```python
from build123d import *

# Parameters (mm, degrees)
BOSS_EXTRUDE1_DEPTH = 2
CUT_EXTRUDE1_REACH  = 186.662
SKETCH3_W           = 25
SKETCH3_H           = 4
CUT_EXTRUDE2_DEPTH  = 185.661853126
SKETCH4_W           = 4
SKETCH4_H           = 10
BOSS_EXTRUDE2_DEPTH = 4


with BuildPart() as part:
    # Sketch1 → Boss-Extrude1 (new, symmetric)
    with BuildSketch(Plane.XY):
        Polygon((0, 4), (0, 72), (-170, 72), (-35, 19), (-35, 4), align=None)
    extrude(amount=BOSS_EXTRUDE1_DEPTH, both=True)

    # Sketch2 → Cut-Extrude1 (cut, up to next)
    with BuildSketch(Plane.XY.offset(2), mode=Mode.PRIVATE) as cut_extrude1_sk1:
        with BuildLine():
            Line((-3, 11), (-3, 7.5))
            ThreePointArc((-3, 7.5), (-4.5, 6), (-6, 7.5))
            Line((-6, 7.5), (-6, 11))
            ThreePointArc((-6, 11), (-4.5, 12.5), (-3, 11))
        make_face()
    cut_extrude1_tool1 = extrude(cut_extrude1_sk1.sketch, amount=-CUT_EXTRUDE1_REACH, mode=Mode.PRIVATE) & part.part
    # Sketch2 → Cut-Extrude1 (cut, up to next)
    with BuildSketch(Plane.XY.offset(2), mode=Mode.PRIVATE) as cut_extrude1_sk2:
        with BuildLine():
            Line((-32, 11), (-32, 7.5))
            ThreePointArc((-32, 7.5), (-30.5, 6), (-29, 7.5))
            Line((-29, 7.5), (-29, 11))
            ThreePointArc((-29, 11), (-30.5, 12.5), (-32, 11))
        make_face()
    cut_extrude1_tool2 = extrude(cut_extrude1_sk2.sketch, amount=-CUT_EXTRUDE1_REACH, mode=Mode.PRIVATE) & part.part
    add(cut_extrude1_tool1.solids().sort_by_distance((-4.5, 9.25, 2))[0], mode=Mode.SUBTRACT)
    add(cut_extrude1_tool2.solids().sort_by_distance((-30.5, 9.25, 2))[0], mode=Mode.SUBTRACT)

    # Sketch3 → Cut-Extrude2 (cut, through all)
    with BuildSketch(Plane.XY.offset(2)):
        with Locations((-62.5, 70)):
            Rectangle(SKETCH3_W, SKETCH3_H)
        with Locations((-12.5, 70)):
            Rectangle(SKETCH3_W, SKETCH3_H)
        with Locations((-112.5, 70)):
            Rectangle(SKETCH3_W, SKETCH3_H)
        with Locations((-162.5, 70)):
            Rectangle(SKETCH3_W, SKETCH3_H)
        with Locations((-212.5, 70)):
            Rectangle(SKETCH3_W, SKETCH3_H)
        with Locations((-262.5, 70)):
            Rectangle(SKETCH3_W, SKETCH3_H)
        with Locations((-312.5, 70)):
            Rectangle(SKETCH3_W, SKETCH3_H)
        with Locations((-362.5, 70)):
            Rectangle(SKETCH3_W, SKETCH3_H)
        with Locations((-412.5, 70)):
            Rectangle(SKETCH3_W, SKETCH3_H)
        with Locations((-462.5, 70)):
            Rectangle(SKETCH3_W, SKETCH3_H)
    extrude(amount=-CUT_EXTRUDE2_DEPTH, mode=Mode.SUBTRACT)

    # Sketch4 → Boss-Extrude2 (add)
    with BuildSketch(Plane(origin=(0, 0, 0), x_dir=(0, 0, -1), z_dir=(1, 0, 0))):
        with Locations((0, 63)):
            Rectangle(SKETCH4_W, SKETCH4_H)
        with Locations((0, 38)):
            Rectangle(SKETCH4_W, SKETCH4_H)
        with Locations((0, 13)):
            Rectangle(SKETCH4_W, SKETCH4_H)
    extrude(amount=BOSS_EXTRUDE2_DEPTH)


solid = part.part
```
Could you check a few things on this model? Use its own coordinates, in mm. A direction names the side the tool comes from. Coordinates: 2 decimals unless noted, no trailing zeros. Loops run counter-clockwise (first coordinate to the right, second up) from the corner with the lowest first, then second, coordinate; pieces in that order, holes last. Notation, with made-up numbers: M 71,2.5 L 119,2.5 A28 cw 119,33.5 Z; hole C -39.5,64 d6. An arc over 180 degrees is marked long. Put each result on its own line as item: value. Start each with the question number.
(1) I need wall thicknesses on line 1 (X direction, y = 9, z = -0.85); line 2 (X direction, y = 69, z = -0.7); line 3 (Y direction, x = -15.5, z = -0.1). Which ranges of each line are inside material? Lowest first, please. Write a range as from..to.
(2) For faces 1 (the face through (-3, 9, 0)), 2 (the face through (0, 6, 0)), 3 (the face through (-50, 70, 0)), 4 (the face through (2, 58, 0)), which set-ups out of +Z, -Z, +X, -X, +Y, -Y let a thin tool reach every point of the face, with its end or its side?
(3) Thinking about a two-plate mould opening in X: for faces 5 (the face through (-4.5, 6, 0)), 6 (the face through (-18, 4, 0)), 7 (the face through (0, 50, 0)), which applies, pulls with the +X half, pulls with the -X half, needs draft (parallel to the pull), parting line crosses it, or undercut?
(4) Will these pins go through, and if not, where does the flat tip stop? P1, Ø2, axis at y = 69.5, z = -0.5, coming from the +X side; P2, Ø2, axis at x = -154.5, z = -1, coming from the +Y side; P3, Ø1.2, axis at y = 70, z = 0.5, coming from the -X side.
(5) Suppose I cut it at C-C on z = 1. Count the separate pieces of the cut face and the enclosed holes in it, then the cut area to 3 significant figures.
(6) Suppose I cut it at D-D on y = 47.5. Please give me the cut outline in (x, z).
(7) Suppose I cut it at A-A on x = -30.5. Please give me the cut outline in (y, z).
(8) Suppose I cut it at B-B on x = -4.5. Please give me the cut outline in (y, z), then the cut area to 3 significant figures.
Solutions:
1. line 1: x = -35..-32, -29..-6, -3..4
1. line 2: x = -150..-125, -100..-75, -50..-25
1. line 3: y = 4..68
2. face 1: +Z, -Z
2. face 2: +Z, -Z, +X, -Y
2. face 3: +Z, -Z, +Y
2. face 4: +Z, -Z, +X
3. face 5: undercut
3. face 6: needs draft
3. face 7: pulls with the +X half
4. P1: stops at x = -25
4. P2: stops at y = 68
4. P3: stops at x = -150
5. separate pieces: 1
5. enclosed holes: 2
5. area: 5,680 mm2
6. outline: M -107.59,-2 L 0,-2 L 0,2 L -107.59,2 Z
7. outline: M 4,-2 L 6,-2 L 6,2 L 4,2 Z; M 12.5,-2 L 72,-2 L 72,2 L 12.5,2 Z
8. outline: M 4,-2 L 6,-2 L 6,2 L 4,2 Z; M 12.5,-2 L 68,-2 L 68,2 L 12.5,2 Z
8. area: 230 mm2
